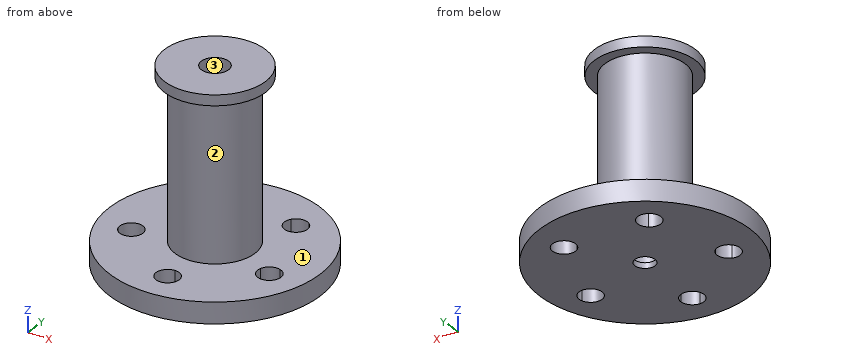
from build123d import *

# Parameters (mm, degrees)
SKETCH1_R           = 31.75
BOSS_EXTRUDE1_DEPTH = 6.35
SKETCH2_R           = 12.065
BOSS_EXTRUDE2_DEPTH = 50.8
BOSS_EXTRUDE3_START = -3.175
SKETCH4_R           = 15.24
SKETCH4_R_2         = 12.065
BOSS_EXTRUDE3_DEPTH = 3.175
CUT_EXTRUDE1_DEPTH  = 68.7994469
CIRPATTERN1_COUNT   = 5
SKETCH6_R           = 3.048
CUT_EXTRUDE2_DEPTH  = 73.679071953
SKETCH6_3_R         = 4.1275
SKETCH6_3_R_2       = 3.048
CUT_EXTRUDE3_DEPTH  = 55.499


with BuildPart() as part:
    # Sketch1 → Boss-Extrude1 (new body)
    with BuildSketch(Plane.XY):
        Circle(SKETCH1_R)
    extrude(amount=BOSS_EXTRUDE1_DEPTH)

    # Sketch2 → Boss-Extrude2 (add)
    with BuildSketch(Plane.XY.offset(6.35)):
        Circle(SKETCH2_R)
    extrude(amount=BOSS_EXTRUDE2_DEPTH)

    # Sketch4 → Boss-Extrude3 (add)
    with BuildSketch(Plane.XY.offset(57.15).offset(BOSS_EXTRUDE3_START)):
        Circle(SKETCH4_R)
        Circle(SKETCH4_R_2, mode=Mode.SUBTRACT)
    extrude(amount=BOSS_EXTRUDE3_DEPTH)

    # Sketch5 → Cut-Extrude1 (cut, through all)
    with BuildSketch(Plane.XY.offset(6.35)):
        with BuildLine():
            ThreePointArc((3.4925, -21.9075), (2.469570433, -19.437929567), (0, -18.415))
            Line((0, -18.415), (0, -25.4))
            ThreePointArc((0, -25.4), (2.469570433, -24.377070433), (3.4925, -21.9075))
        make_face()
        with BuildLine():
            Line((0, -25.4), (0, -18.415))
            ThreePointArc((0, -18.415), (-3.4925, -21.9075), (0, -25.4))
        make_face()
    cut_extrude1 = extrude(amount=-CUT_EXTRUDE1_DEPTH, mode=Mode.SUBTRACT)

    # CirPattern1: Cut-Extrude1 ×5 about axis
    cirpattern1_axis = Axis((0, 0, 0), (0, 0, 1))
    for i in range(1, CIRPATTERN1_COUNT):
        add(cut_extrude1.rotate(cirpattern1_axis, i * 360 / CIRPATTERN1_COUNT), mode=Mode.SUBTRACT)

    # Sketch6 → Cut-Extrude2 (cut, through all)
    with BuildSketch(Plane.XY.offset(57.15)):
        Circle(SKETCH6_R)
    extrude(amount=-CUT_EXTRUDE2_DEPTH, mode=Mode.SUBTRACT)

    # Sketch6_3 → Cut-Extrude3 (cut)
    with BuildSketch(Plane.XY.offset(57.15)):
        Circle(SKETCH6_3_R)
        Circle(SKETCH6_3_R_2, mode=Mode.SUBTRACT)
    extrude(amount=-CUT_EXTRUDE3_DEPTH, mode=Mode.SUBTRACT)


solid = part.part
Can you work these out from the model? Positions are in its coordinate system, mm. Face numbers are marked on the shaded views. Coordinates: 2 decimals unless noted, no trailing zeros. Write each loop counter-clockwise with the first axis right and the second up, starting at its lowest first coordinate (ties: lowest second). Pieces come first, ordered by that corner, then holes. Notation, with made-up numbers: (32, 82.5) -> (48, 82.5) arc R9 cw to (48, 92.5) -> close; hole circle Ø7 at (-11, -19). An arc over 180 degrees is marked (long way). Answer as CSV lines item,"result".
1) If we mould it in two halves opening along Y, with no side actions, what happens to the marked faces 1, 2 and 3? For each: +Y half, -Y half, draft (parallel to the pull), parting line (faces both ways), or undercut.
Check result:
face 1,"draft"
face 2,"parting line"
face 3,"undercut"
2) If I drill on line 1 (Y direction, x = 0, z = 18) (1 decimal); line 2 (Z direction, x = -10, y = 11) (3 decimals); line 3 (Z direction, x = -17, y = 6), over which ranges is the centre line in solid material (lowest first)? Write a range as from..to.
Check result:
line 1,"-12.1..-4.1, 4.1..12.1"
line 2,"0..6.35, 53.975..57.15"
line 3,"0..6.35"
3) If we section it at B-B on z = 37.5: Please give me the cut outline in (x, y) (1 decimal).
Check result:
outline,"circle Ø24.1 at (0, 0); hole circle Ø8.3 at (0, 0)"
4) If we section it at C-C on x = 1: Please give me the cut outline in (y, z) (3 decimals).
Check result:
outline,"(-31.734, 0) -> (-25.254, 0) -> (-25.254, 6.35) -> (-31.734, 6.35) -> close; (-18.561, 0) -> (-2.879, 0) -> (-2.879, 1.651) -> (-4.005, 1.651) -> (-4.005, 57.15) -> (-15.207, 57.15) -> (-15.207, 53.975) -> (-12.023, 53.975) -> (-12.023, 6.35) -> (-18.561, 6.35) -> close; (2.879, 0) -> (31.734, 0) -> (31.734, 6.35) -> (12.023, 6.35) -> (12.023, 53.975) -> (15.207, 53.975) -> (15.207, 57.15) -> (4.005, 57.15) -> (4.005, 1.651) -> (2.879, 1.651) -> close"
5) If we section it at D-D on x = -7: Please give me the cut outline in (y, z) (3 decimals).
Check result:
outline,"(-30.969, 0) -> (30.969, 0) -> (30.969, 6.35) -> (9.827, 6.35) -> (9.827, 53.975) -> (13.537, 53.975) -> (13.537, 57.15) -> (-13.537, 57.15) -> (-13.537, 53.975) -> (-9.827, 53.975) -> (-9.827, 6.35) -> (-30.969, 6.35) -> close"
6) Will these pins go through, and if not, where does the flat tip stop? P1, Ø1.5, axis at y = -11.5, z = 43, coming from the +X side; P2, Ø10, axis at x = 18.5, y = 22, coming from the +Z side; P3, Ø4, axis at y = 9, z = 37.5, coming from the -X side; P4, Ø5, axis at x = 0, y = 0, coming from the -Z side.
Check result:
P1,"x = 5.48"
P2,"z = 6.35"
P3,"x = -9.83"
P4,"through"
